The model under review builds one solid part; all positions refer to its coordinate system, in mm. Face numbers are marked on the shaded views. Give positions to 0.01 mm unless a question says otherwise; leave off trailing zeros. Write each loop counter-clockwise with the first axis right and the second up, starting at its lowest first coordinate (ties: lowest second). Pieces come first, ordered by that corner, then holes.
from build123d import *

# Parameters (mm, degrees)
SKETCH1_R           = 0.95
SKETCH1_R_2         = 1.25
BOSS_EXTRUDE1_DEPTH = 3
SKETCH2_R           = 2.169910798
BOSS_EXTRUDE2_DEPTH = 13
CHAMFER1_SIZE       = 1.2


with BuildPart() as part:
    # Sketch1 → Boss-Extrude1 (new body)
    with BuildSketch(Plane(origin=(0, 0, 0), x_dir=(1, 0, 0), z_dir=(0, 1, 0))):
        with BuildLine():
            ThreePointArc((2.227105745, 2.7), (-3.5, 0), (2.227105745, -2.7))
            Line((2.227105745, -2.7), (16.12932144, -1.193011301))
            ThreePointArc((16.12932144, -1.193011301), (17.2, 0), (16.12932144, 1.193011301))
            Line((16.12932144, 1.193011301), (2.227105745, 2.7))
        make_face()
        with Locations(Location((12.5, 0, 0), (0, 0, 270))):
            Circle(SKETCH1_R, mode=Mode.SUBTRACT)
        with Locations(Location((0, 0, 0), (0, 0, 270))):
            Circle(SKETCH1_R_2, mode=Mode.SUBTRACT)
    extrude(amount=BOSS_EXTRUDE1_DEPTH)

    # Sketch2 → Boss-Extrude2 (add)
    with BuildSketch(Plane(origin=(0, 3, 0), x_dir=(1, 0, 0), z_dir=(0, 1, 0))):
        with Locations(Location((7, 0, 0), (0, 0, 83.813341225))):
            Circle(SKETCH2_R)
    extrude(amount=BOSS_EXTRUDE2_DEPTH)

    # Chamfer1
    # the kernel refuses this chamfer: 1.2 mm, written as the material it adds along each edge
    with BuildSketch(Plane(origin=(7, 3, 0), x_dir=(0.1077678664159532, 0, -0.9941760844881318), z_dir=(0.9941760844881318, 0, 0.1077678664159532))) as chamfer1_piece_1_section:
        Polygon((2.169910798 + CHAMFER1_SIZE, 0), (2.169910798, CHAMFER1_SIZE), (2.169910798, 0), align=None)
    chamfer1_piece_1 = revolve(axis=Axis((7, 3, 0), (0, 1, 0)), revolution_arc=192.373317929, mode=Mode.PRIVATE)
    chamfer1_piece_1 = split(chamfer1_piece_1, bisect_by=Plane(origin=(4.507411797, 3.588560711, 2.452816707), z_dir=(-0.10776786640872232, 0, -0.9941760844889158)), keep=Keep.TOP, mode=Mode.PRIVATE)
    chamfer1_piece_1 = split(chamfer1_piece_1, bisect_by=Plane(origin=(4.507411799, 3.588560711, -2.452816707), z_dir=(-0.10776786640872232, 0, 0.9941760844889158)), keep=Keep.TOP, mode=Mode.PRIVATE)
    add(chamfer1_piece_1)
    with BuildSketch(Plane(origin=(7, 3, 0), x_dir=(0.1077678729849121, 0, 0.9941760837760621), z_dir=(-0.9941760837760621, 0, 0.1077678729849121))) as chamfer1_piece_2_section:
        Polygon((2.169910798 + CHAMFER1_SIZE, 0), (2.169910798, CHAMFER1_SIZE), (2.169910798, 0), align=None)
    chamfer1_piece_2 = revolve(axis=Axis((7, 3, 0), (0, 1, 0)), revolution_arc=167.626682071, mode=Mode.PRIVATE)
    chamfer1_piece_2 = split(chamfer1_piece_2, bisect_by=Plane(origin=(9.961043045, 3.589331186, 1.861647585), z_dir=(-0.10776786640872232, 0, -0.9941760844889158)), keep=Keep.TOP, mode=Mode.PRIVATE)
    chamfer1_piece_2 = split(chamfer1_piece_2, bisect_by=Plane(origin=(9.961043043, 3.589331186, -1.861647585), z_dir=(-0.10776786640872232, 0, 0.9941760844889158)), keep=Keep.TOP, mode=Mode.PRIVATE)
    add(chamfer1_piece_2)


solid = part.part
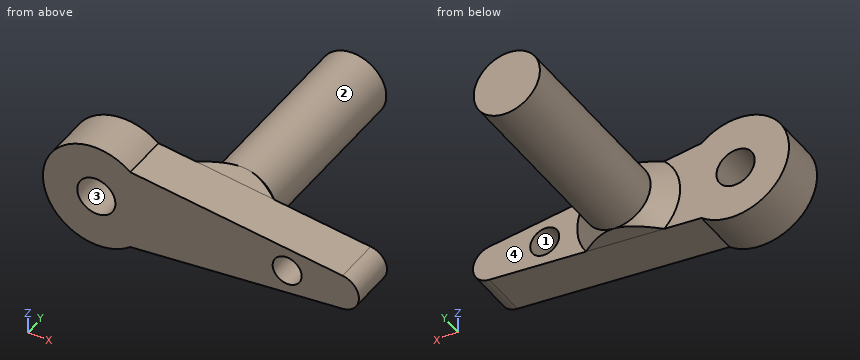
1) Insertion check: pin 1 (3 mm diameter, centred on x = 14, z = 1, fed in from +Y); pin 2 (4 mm diameter, centred on y = 2.5, z = 2.5, fed in from -X); pin 3 (8 mm diameter, centred on x = 7, y = 5.5, fed in from -Z); pin 4 (1.5 mm diameter, centred on x = 0, z = 0, fed in from +Y). Each pin has a flat end and moves straight along its axis. Give the tip position at first contact, or say it passes through.
2) The part is to be moulded in two halves that separate along Z. For the marked faces 1, 2, 3 and 4, say which applies: +Z half, -Z half, draft (parallel to the pull), parting line (faces both ways), or undercut.
3) Consider section D-D, the plane x = 12.5. Give the boundary of the cut face in (y, z).
4) To check wall thickness, follow probe 1 along X at (y, z) = (1.25, 0.75); probe 2 along Y at (x, z) = (10, 1.75); probe 3 along X at (y, z) = (4.5, 0.25). State the ranges of each line that lie inside material, in increasing order.
5) Consider section B-B, the plane z = 0. Give the boundary of the cut face in (x, y), then the cut area to 3 significant figures.
6) Consider section C-C, the plane y = 2. Give the boundary of the cut face in (x, z), then the cut area to 3 significant figures.
7) Consider section A-A, the plane x = 0. Give the boundary of the cut face in (y, z).
Answer block:
1. pin 1: stops at y = 3
1. pin 2: stops at x = -3.46
1. pin 3: stops at z = -2.52
1. pin 4: passes through
2. face 1: undercut
2. face 2: parting line
2. face 3: undercut
2. face 4: draft
3. outline: (0, -1.59) - (3, -1.59) - (3, -0.95) - (0, -0.95) - close; (0, 0.95) - (3, 0.95) - (3, 1.59) - (0, 1.59) - close
4. probe 1: x = -3.42 to -1, 1 to 11.92, 13.08 to 16.94
4. probe 2: y = 0 to 3
4. probe 3: x = 4.84 to 9.16
5. outline: (-3.5, 0) - (-1.25, 0) - (-1.25, 3) - (-3.5, 3) - close; (1.25, 0) - (11.55, 0) - (11.55, 3) - (10.37, 3) - (9.17, 4.2) - (9.17, 16) - (4.83, 16) - (4.83, 4.2) - (3.63, 3) - (1.25, 3) - close; (13.45, 0) - (17.2, 0) - (17.2, 3) - (13.45, 3) - close
5. area: 107 mm2
6. outline: (2.23, -2.7) - (16.13, -1.19) arc R1.2 ccw to (16.13, 1.19) - (2.23, 2.7) arc R3.5 ccw (long way) to start; hole circle Ø2.5 at (0, 0); hole circle Ø1.9 at (12.5, 0)
6. area: 82.0 mm2
7. outline: (0, -3.5) - (3, -3.5) - (3, -1.25) - (0, -1.25) - close; (0, 1.25) - (3, 1.25) - (3, 3.5) - (0, 3.5) - close
